For this review, take the finished solid that the model builds, in its own axes (mm). Coordinates: 2 decimals unless noted, no trailing zeros. Loops run counter-clockwise (first coordinate to the right, second up) from the corner with the lowest first, then second, coordinate; pieces in that order, holes last. Notation, with made-up numbers: (82, 18.5) - (92, 18.5) arc R18 ccw to (92, 28.5) - close; hole circle Ø4 at (-20.75, 47.5). An arc over 180 degrees is marked (long way). Answer as a JSON object with one key per item and string values. Group by question number.
Item 1: We need section A-A (x = -45). Give the boundary of the cut face in (y, z).
Item 2: Clearance check with flat-ended pins moving along their axes: pin 1 (1 mm diameter, centred on y = 1, z = -21, fed in from +X); pin 2 (1.9 mm diameter, centred on x = -45, z = -10.43, fed in from -Y); pin 3 (0.9 mm diameter, centred on x = -22.5, y = 2, fed in from -Z). State where each tip first meets the part, or that it passes through.
Item 3: We need section B-B (y = 0.7). Give the boundary of the cut face in (x, z), then the cut area to 3 significant figures.
Item 4: To check wall thickness, follow line 1 (Z direction, x = -51.5, y = 0.8); line 2 (X direction, y = 2.7, z = -22); line 3 (X direction, y = 1.05, z = -7). State the ranges of each line that lie inside material, in increasing order.
Item 5: We need section D-D (z = -14.5). Give the boundary of the cut face in (x, y).
Item 6: We need section C-C (x = -33). Give the boundary of the cut face in (y, z), then the cut area to 3 significant figures.
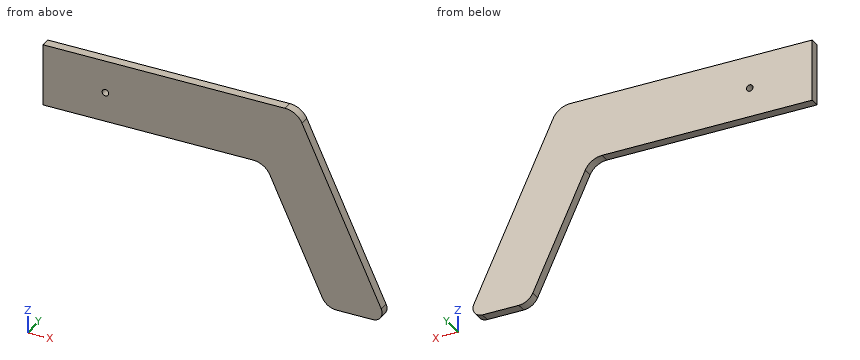
from build123d import *

# Parameters (mm, degrees)
ESBO_O1_R                = 1.05
RESSALTO_EXTRUS_O1_DEPTH = 3


with BuildPart() as part:
    # Esboço1 → Ressalto-extrusão1 (new body)
    with BuildSketch(Plane(origin=(0, 0, 0), x_dir=(1, 0, 0), z_dir=(0, 1, 0))):
        with BuildLine():
            Line((-65, 19.865476825), (-65, 0))
            Line((-65, 0), (0, 0))
            Line((0, 0), (12.574875441, 0))
            ThreePointArc((12.574875441, 0), (15.798673091, 0.939651325), (18.012722163, 3.46429043))
            Line((18.012722163, 3.46429043), (43.410601428, 57.93021828))
            ThreePointArc((43.410601428, 57.93021828), (43.221852405, 60.80997189), (40.691678067, 62.198073065))
            Line((40.691678067, 62.198073065), (29.011685815, 62.198073065))
            ThreePointArc((29.011685815, 62.198073065), (26.348436448, 61.421806665), (24.519362347, 59.336147382))
            Line((24.519362347, 59.336147382), (7.729311551, 23.329767255))
            ThreePointArc((7.729311551, 23.329767255), (5.515262479, 20.80512815), (2.291464829, 19.865476825))
            Line((2.291464829, 19.865476825), (-65, 19.865476825))
        make_face()
        with Locations(Location((-45, 10.43351307, 0), (0, 0, 270))):
            Circle(ESBO_O1_R, mode=Mode.SUBTRACT)
    extrude(amount=RESSALTO_EXTRUS_O1_DEPTH)


solid = part.part
Check sheet entries:
{
 "1": {"outline": "(0, -19.87) - (3, -19.87) - (3, -11.48) - (0, -11.48) - close; (0, -9.38) - (3, -9.38) - (3, 0) - (0, 0) - close"},
 "2": {"pin 1": "stops at x = 26.42", "pin 2": "passes through", "pin 3": "stops at z = -19.87"},
 "3": {"outline": "(-65, -19.87) - (2.29, -19.87) arc R6 cw to (7.73, -23.33) - (24.52, -59.34) arc R4.96 ccw to (29.01, -62.2) - (40.69, -62.2) arc R3 ccw to (43.41, -57.93) - (18.01, -3.46) arc R6 ccw to (12.57, 0) - (-65, 0) - close; hole circle Ø2.1 at (-45, -10.43)", "area": "2,530 mm2"},
 "4": {"line 1": "z = -19.87 to 0", "line 2": "x = 6.88 to 26.66", "line 3": "x = -65 to 19.66"},
 "5": {"outline": "(-65, 0) - (23.16, 0) - (23.16, 3) - (-65, 3) - close"},
 "6": {"outline": "(0, -19.87) - (3, -19.87) - (3, 0) - (0, 0) - close", "area": "59.6 mm2"}
}
